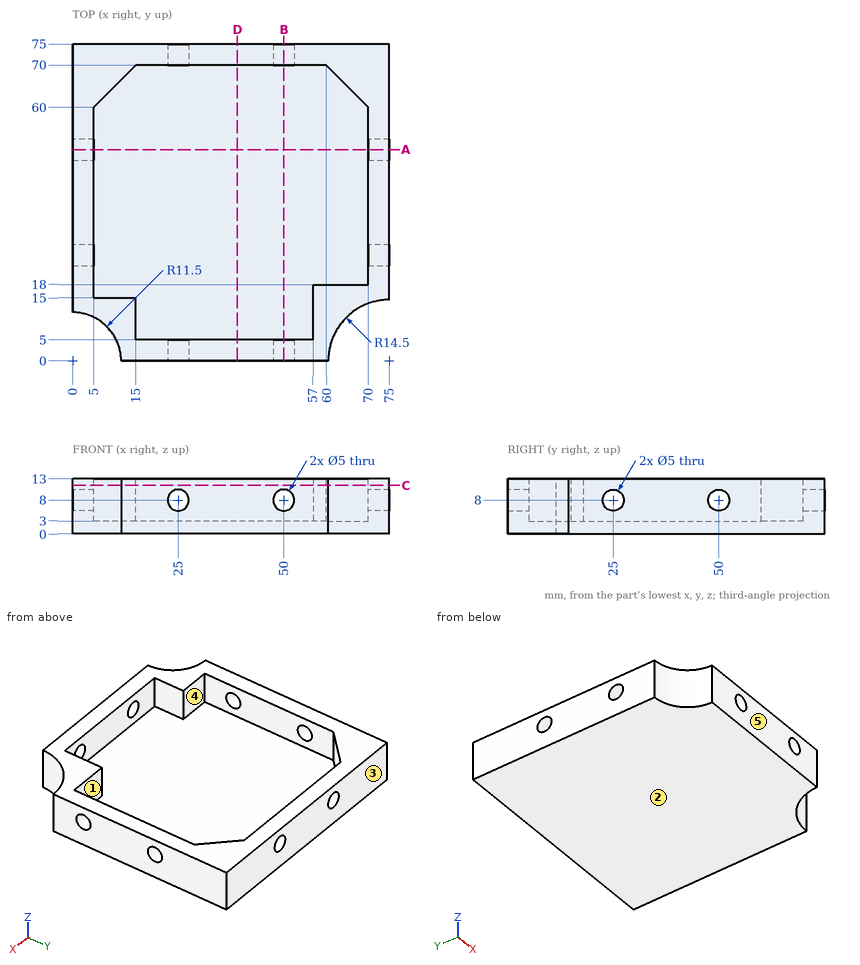
Source: three-view drawing plus pictorial views. Frame: mm from the lowest corner of the part. A direction names the side the tool comes from. Give positions to 0.01 mm unless a question says otherwise; leave off trailing zeros. Order: outer loops, then holes, each group sorted by start corner. A loop starts at its lowest first (then second) coordinate and runs counter-clockwise, first axis right, second up. Notation, with made-up numbers: (-37.75, 21) - (5.25, 21) arc R16 cw to (5.25, 33) - close; hole circle Ø9 at (82, 75.5). An arc over 180 degrees is marked (long way). Answer as a JSON object with one key per item and string values. Group by question number.
Q1. Mould query, pull axis Y, two halves, no side actions, for the marked faces 1, 2 and 3. Classes: pulls with the +Y half, pulls with the -Y half, needs draft (parallel to the pull), parting line crosses it, or undercut.
Q2. First-contact query: pin 1 Ø6 at (y, z) = (42.5, 10.5) entering from -X; pin 2 Ø19.5 at (x, y) = (38.5, 45) entering from +Z. Flat tips, straight axial feed; report the tip coordinate or a pass-through.
Q3. Line query: probe 1 along X at (y, z) = (71.45, 8); probe 2 along X at (y, z) = (22.5, 7); probe 3 along Z at (x, y) = (72.85, 50). Output: solid intervals per line, ascending.
Q4. Cut plane A-A, the plane y = 50. Output: boundary loops of the cut face in (x, z), then the cut area to 3 significant figures.
Q5. Cut plane C-C, the plane z = 11.5. Output: boundary loops of the cut face in (x, y).
Q6. Cut plane D-D, the plane x = 39. Output: boundary loops of the cut face in (y, z), then the cut area to 3 significant figures.
Q7. Set-up query: the marked faces 4 and 5. Return all of +Z, -Z, +X, -X, +Y, -Y with unobstructed straight access to the full face (end or side cutting, diameter ignored); none if empty.
Results:
{
 "1": {"face 1": "undercut", "face 2": "needs draft", "face 3": "pulls with the +Y half"},
 "2": {"pin 1": "x = 0", "pin 2": "z = 3"},
 "3": {"probe 1": "0 to 22.5, 27.5 to 47.5, 52.5 to 75", "probe 2": "0 to 5, 70 to 75", "probe 3": "0 to 5.5, 10.5 to 13"},
 "4": {"outline": "(0, 0) - (75, 0) - (75, 5.5) - (70, 5.5) - (70, 3) - (5, 3) - (5, 5.5) - (0, 5.5) - close; (0, 10.5) - (5, 10.5) - (5, 13) - (0, 13) - close; (70, 10.5) - (75, 10.5) - (75, 13) - (70, 13) - close", "area": "275 mm^2"},
 "5": {"outline": "(0, 11.5) arc R11.5 cw to (11.5, 0) - (60.5, 0) arc R14.5 cw to (75, 14.5) - (75, 75) - (0, 75) - close; hole (5, 15) - (15, 15) - (15, 5) - (57, 5) - (57, 18) - (70, 18) - (70, 60) - (60, 70) - (15, 70) - (5, 60) - close"},
 "6": {"outline": "(0, 0) - (75, 0) - (75, 13) - (70, 13) - (70, 3) - (5, 3) - (5, 13) - (0, 13) - close", "area": "325 mm^2"},
 "7": {"face 4": "+Z", "face 5": "+Z, -Z, +X, -X, -Y"}
}
